The model under review builds one solid part; all positions refer to its coordinate system, in mm. A direction names the side the tool comes from. Round coordinates to 2 decimals unless told otherwise and drop trailing zeros. Order: outer loops, then holes, each group sorted by start corner. A loop starts at its lowest first (then second) coordinate and runs counter-clockwise, first axis right, second up. Notation, with made-up numbers: M 31,47.25 L 81,47.25 A19 cw 81,60.25 Z; hole C 8,-33 d1. An arc over 180 degrees is marked long. One line per item, written item: value. Start each with the question number.
from build123d import *

# Parameters (mm, degrees)
BOSS_EXTRUDE1_DEPTH                              = 119.888
CBORE_FOR_1_4_SOCKET_HEAD_CAP_SCREW1_D           = 6.7564
CBORE_FOR_1_4_SOCKET_HEAD_CAP_SCREW1_CBORE_D     = 11.1125
CBORE_FOR_1_4_SOCKET_HEAD_CAP_SCREW1_CBORE_DEPTH = 6.35
SKETCH4_R                                        = 5.715
CUT_EXTRUDE1_DEPTH                               = 124.034883785
BOSS_EXTRUDE2_DEPTH                              = 2.54
LPATTERN1_COUNT                                  = 2
LPATTERN1_PITCH                                  = 27.2542
LPATTERN1_COL_COUNT                              = 2
LPATTERN1_COL_PITCH                              = 27.2542
SKETCH6_R                                        = 9.525
CUT_EXTRUDE2_DEPTH                               = 2.54


with BuildPart() as part:
    # Sketch1 → Boss-Extrude1 (new body)
    with BuildSketch(Plane(origin=(0, 0, 0), x_dir=(1, 0, 0), z_dir=(0, 1, 0))):
        Polygon((0, 0), (0, 10.922), (-25.4, 10.922), (-25.4, 7.5565), (-21.155673935, 0), align=None)
    extrude(amount=BOSS_EXTRUDE1_DEPTH)

    # CBORE for 1/4 Socket Head Cap Screw1 (through all)
    with Locations(Plane(origin=(0, 0, -10.922), x_dir=(-1, 0, 0), z_dir=(0, 0, -1))):
        with Locations((12.7, 109.77245), (12.7, 10.11555)):
            CounterBoreHole(CBORE_FOR_1_4_SOCKET_HEAD_CAP_SCREW1_D / 2, CBORE_FOR_1_4_SOCKET_HEAD_CAP_SCREW1_CBORE_D / 2, CBORE_FOR_1_4_SOCKET_HEAD_CAP_SCREW1_CBORE_DEPTH)

    # Sketch4 → Cut-Extrude1 (cut, through all)
    with BuildSketch(Plane(origin=(0, 0, -10.922), x_dir=(-1, 0, 0), z_dir=(0, 0, -1))):
        with Locations((0, 59.944)):
            Circle(SKETCH4_R)
    extrude(amount=-CUT_EXTRUDE1_DEPTH, mode=Mode.SUBTRACT)

    # Sketch5 → Boss-Extrude2 (add, symmetric)
    with BuildSketch(Plane(origin=(0, 59.944, 0), x_dir=(1, 0, 0), z_dir=(0, 1, 0))):
        Polygon((-21.155673935, 0), (-20.157008978, -1.778), (-13.045008978, -1.778), (-12.046344022, 0), align=None)
    boss_extrude2 = extrude(amount=BOSS_EXTRUDE2_DEPTH, both=True)

    # LPattern1: Boss-Extrude2 ×2
    with Locations(*[(0, -i * LPATTERN1_PITCH, 0) for i in range(1, LPATTERN1_COUNT)]):
        add(boss_extrude2)

    # LPattern1 col: Boss-Extrude2 ×2
    with Locations(*[(0, i * LPATTERN1_COL_PITCH, 0) for i in range(1, LPATTERN1_COL_COUNT)]):
        add(boss_extrude2)

    # Sketch6 → Cut-Extrude2 (cut)
    with BuildSketch(Plane.XY):
        with Locations((0, 59.944)):
            Circle(SKETCH6_R)
    extrude(amount=-CUT_EXTRUDE2_DEPTH, mode=Mode.SUBTRACT)


solid = part.part
Item 1: Wall thickness on L1, parallel to Y at x = -12.7, z = -6; L2, parallel to Y at x = -12.7, z = -2.85; L3, parallel to Z at x = -10.75, y = 28: over which ranges is each line inside the solid? List them lowest first.
Item 2: Clearance check with flat-ended pins moving along their axes: P1, Ø0.9, axis at x = -16, z = 0.5, coming from the +Y side; P2, Ø4, axis at x = -5, y = 65, coming from the +Z side; P3, Ø3, axis at y = 57, z = -8.5, coming from the +X side. State where each tip first meets the part, or that it passes through.
Item 3: The part is to be moulded in two halves that separate along X. For faces 1 (the flat face through (-17, 33, 1.778)), 2 (the cylindrical face through (-13.14, 13.465, -2.254)), 3 (the flat face through (-25.4, 59, -9)), 4 (the flat face through (-13, 6, -4.572)), say which applies: pulls with the +X half, pulls with the -X half, needs draft (parallel to the pull), parting line crosses it, or undercut.
Item 4: Consider section B-B, the plane z = -9.75. Give the boundary of the cut face in (x, y) (1 decimal).
Item 5: Machinability: for faces 5 (the cylindrical face through (-5.714, 59.818, -6.79)), 6 (the cylindrical face through (-11.98, 115.28, -7.79)), 7 (the flat face through (-6, 60, -2.54)), which of the approach directions +Z, -Z, +X, -X, +Y, -Y give a long, thin tool a straight path to every point of the face, cutting with its end or side? Answer none if there is none.
Item 6: Consider section A-A, the plane y = 80. Give the boundary of the cut face in (x, z), then the cut area to 3 significant figures.
Item 7: Consider section C-C, the plane y = 55.5. Give the boundary of the cut face in (x, z).
Computed:
1. L1: y = 0 to 4.56, 15.67 to 104.22, 115.33 to 119.89
1. L2: y = 0 to 6.74, 13.49 to 106.39, 113.15 to 119.89
1. L3: z = -10.92 to 0
2. P1: stops at y = 89.74
2. P2: stops at z = -2.54
2. P3: stops at x = -3.59
3. face 1: needs draft
3. face 2: undercut
3. face 3: pulls with the -X half
3. face 4: undercut
4. outline: M -25.4,0 L 0,0 L 0,54.2 A5.7 cw 0,65.7 L 0,119.9 L -25.4,119.9 Z; hole C -12.7,10.1 d11.1; hole C -12.7,109.8 d11.1
5. face 5: +Z, -Z, +X
5. face 6: -Z
5. face 7: +Z, +X
6. outline: M -25.4,-10.92 L 0,-10.92 L 0,0 L -21.16,0 L -25.4,-7.56 Z
6. area: 261 mm^2
7. outline: M -25.4,-10.92 L -3.59,-10.92 L -3.59,-2.54 L -8.42,-2.54 L -8.42,0 L -21.16,0 L -25.4,-7.56 Z
